from build123d import *

# Parameters (mm, degrees)
F0_W      = 9.647341
F0_H      = 3.250734
F2_DEPTH  = 12.7
F4_DEPTH  = 1.778
F5_DEPTH  = 0.508
F1_W      = 1.800112
F1_H      = 1.303531
F6_DEPTH  = 0.381
F1_W_2    = 1.769075
F7_DEPTH  = 0.381
F9_DEPTH  = 3.81
F10_DEPTH = 16.51
F12_DEPTH = 1.016
F13_DEPTH = 0.762


with BuildPart() as f2:
    # F0 (on Front) → F2 (new body)
    with BuildSketch(Plane.XZ):
        with Locations((4.82367, 1.625367)):
            Rectangle(F0_W, F0_H)
        Polygon((-1.701648, 3.250734), (0, 3.250734), (9.647341, 3.250734), (11.377569, 3.250734), (11.377569, 30.514956), (11.391672, 30.514956), (11.391672, 46.697617), (-1.701648, 46.697617), (-1.701648, 30.514956), align=None)
    extrude(amount=F2_DEPTH)

    # F1 (on face) → F4 (join)
    with BuildSketch(Plane.XZ):
        Polygon((3.710789, 33.669334), (3.710789, 30.938132), (6.255776, 30.938132), (6.255776, 33.669334), (6.255776, 34.972865), (6.255776, 36.772978), (3.710789, 36.772978), (3.710789, 34.972865), align=None)
    extrude(amount=-F4_DEPTH)

    # F1 (on face) → F5 (join)
    with BuildSketch(Plane.XZ):
        Polygon((1.855394, 38.511015), (3.710789, 38.511015), (6.255776, 38.511015), (8.024851, 38.511015), (9.793927, 38.511015), (9.793927, 40.124908), (0, 40.124908), (0, 38.511015), align=None)
    extrude(amount=-F5_DEPTH)

    # F1 (on face) → F6 (join)
    with BuildSketch(Plane.XZ):
        with Locations((2.810733, 34.3211)):
            Rectangle(F1_W, F1_H)
    extrude(amount=-F6_DEPTH)

    # F1 (on face) → F7 (join)
    with BuildSketch(Plane.XZ):
        with Locations((7.140313, 34.3211)):
            Rectangle(F1_W_2, F1_H)
    extrude(amount=-F7_DEPTH)

    # F8 (on face) → F9 (join)
    with BuildSketch(Plane.YZ.offset(11.377569)):
        Polygon((0, 27.125444), (-3.33655, 30.514956), (-3.445342, 30.514956), (-6.820974, 27.192068), (0, 20.262824), align=None)
        Polygon((4.431088, 22.624021), (0, 27.125444), (0, 20.262824), (1.000203, 19.246745), align=None)
    extrude(amount=F9_DEPTH)

    # F8 (on face) → F10 (join)
    with BuildSketch(Plane.YZ.offset(11.377569)):
        Polygon((4.431088, 22.624021), (-3.39009, 30.569345), (-6.820974, 27.192068), (1.000203, 19.246745), align=None)
    extrude(amount=-F10_DEPTH)

    # F11 (on face) → F12 (join)
    with BuildSketch(Plane.XZ):
        Polygon((0, 33.361174), (-1.701648, 33.361174), (-1.701648, 30.514956), (-1.701648, 27.172441), (11.316204, 27.172441), (11.316204, 33.361174), (10.014145, 33.361174), (10.014145, 32.268375), (10.014145, 31.780105), (8.293568, 31.780105), (8.293568, 30.268786), (6.968258, 30.268786), (6.968258, 28.431954), (3.108585, 28.431954), (3.108585, 30.268786), (1.899531, 30.268786), (1.899531, 31.780105), (0, 31.780105), (0, 32.268375), align=None)
    extrude(amount=-F12_DEPTH)

    # F11 (on face) → F13 (join)
    with BuildSketch(Plane.XZ):
        Polygon((2.341301, 32.268375), (0, 32.268375), (0, 31.780105), (1.899531, 31.780105), (1.899531, 30.268786), (3.108585, 30.268786), (3.108585, 28.431954), (6.968258, 28.431954), (6.968258, 30.268786), (8.293568, 30.268786), (8.293568, 31.780105), (10.014145, 31.780105), (10.014145, 32.268375), (7.8983, 32.268375), (7.8983, 30.640803), (6.34048, 30.640803), (6.34048, 29.361997), (3.66661, 29.361997), (3.66661, 30.617552), (2.341301, 30.617552), align=None)
    extrude(amount=-F13_DEPTH)


solid = f2.part
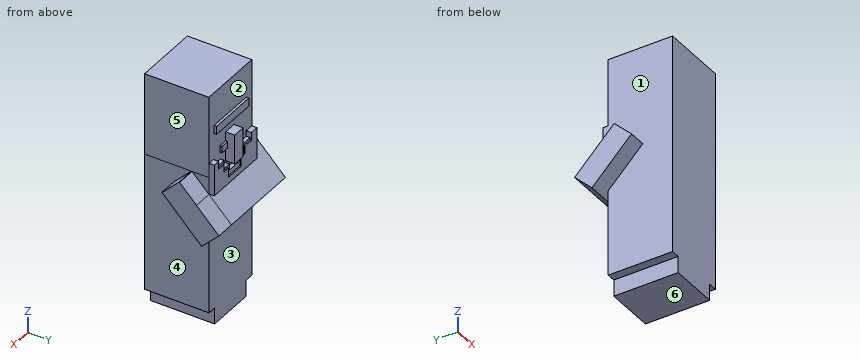
The listing builds one solid part. Answer for the finished solid, in the listing's coordinates (mm). Face numbers are marked on the shaded views. A direction names the side the tool comes from. Round coordinates to 2 decimals unless told otherwise and drop trailing zeros. Order: outer loops, then holes, each group sorted by start corner. A loop starts at its lowest first (then second) coordinate and runs counter-clockwise, first axis right, second up. Notation, with made-up numbers: (-33.75, 67) - (17.25, 67) arc R18 cw to (17.25, 96) - close; hole circle Ø4 at (61.5, 85). An arc over 180 degrees is marked (long way). Write item = value, one per line. Start each with the question number.
1) Section A-A, the plane x = 5.5 is taken. Write down the section's boundary in (y, z).
2) Section C-C, the plane x = 0.5 is taken. Write down the section's boundary in (y, z), plus the area to 3 significant figures.
3) Given pin 1 (4 mm diameter, centred on x = 5, z = 35.5, fed in from +Y); pin 2 (1.9 mm diameter, centred on x = 2, z = 29.5, fed in from +Y); pin 3 (1 mm diameter, centred on x = 10.5, y = -3, fed in from -Z), each flat-ended and moving along its own axis, determine where each tip first touches the part or whether it passes through.
4) For the marked faces 5 and 6, determine the directions among +Z, -Z, +X, -X, +Y, -Y from which every point of the face is accessible in a straight line to the end or side of a thin tool.
5) For a pull along X with two mould halves and no side action, classify the marked faces 1, 2, 3 and 4 as released by +X, released by -X, zero draft, split by the parting line, or undercut.
6) Section B-B, the plane z = 39 is taken. Write down the section's boundary in (x, y).
7) Section D-D, the plane z = 15 is taken. Write down the section's boundary in (x, y).
8) Straight lines are drawn through the part: L1, parallel to Z at x = -1.5, y = -2; L2, parallel to X at y = -4, z = 17.5; L3, parallel to Y at x = 4.75, z = 8. For each, find the intervals that lie inside material, in ascending order.
Results list:
q1.outline = (-12.7, 0) - (0, 0) - (0, 20.26) - (1, 19.25) - (4.43, 22.62) - (0, 27.13) - (0, 27.17) - (1.02, 27.17) - (1.02, 28.43) - (0.76, 28.43) - (0.76, 29.36) - (0, 29.36) - (0, 30.94) - (1.78, 30.94) - (1.78, 36.77) - (0, 36.77) - (0, 38.51) - (0.51, 38.51) - (0.51, 40.12) - (0, 40.12) - (0, 46.7) - (-12.7, 46.7) - close
q2.outline = (-12.7, 0) - (0, 0) - (0, 20.26) - (1, 19.25) - (4.43, 22.62) - (0, 27.13) - (0, 27.17) - (1.02, 27.17) - (1.02, 31.78) - (0.76, 31.78) - (0.76, 32.27) - (0, 32.27) - (0, 38.51) - (0.51, 38.51) - (0.51, 40.12) - (0, 40.12) - (0, 46.7) - (-12.7, 46.7) - close
q2.area = 618 mm^2
q3.pin_1 = 1.78
q3.pin_2 = 1.02
q3.pin_3 = 3.25
q4.face_5 = +Z, +X, +Y, -Y
q4.face_6 = -Z, +X, -X, +Y, -Y
q5.face_1 = released by -X
q5.face_2 = undercut
q5.face_3 = zero draft
q5.face_4 = released by +X
q6.outline = (-1.7, -12.7) - (11.39, -12.7) - (11.39, 0) - (9.79, 0) - (9.79, 0.51) - (0, 0.51) - (0, 0) - (-1.7, 0) - close
q7.outline = (-1.7, -12.7) - (11.38, -12.7) - (11.38, 0) - (-1.7, 0) - close
q8.L1 = 3.25 to 46.7
q8.L2 = -1.7 to 11.38
q8.L3 = -12.7 to 0
